Here's how the part is built. I have some questions about the finished solid (model axes, mm). Face numbers are marked on the shaded views. A direction names the side the tool comes from. Coordinates: 2 decimals unless noted, no trailing zeros. Order: outer loops, then holes, each group sorted by start corner. A loop starts at its lowest first (then second) coordinate and runs counter-clockwise, first axis right, second up. Notation, with made-up numbers: (-4, -3.5) - (37, -3.5) arc R20 cw to (37, 4.5) - close; hole circle Ø6 at (-20.5, -8.75). An arc over 180 degrees is marked (long way). Answer as CSV lines item,"result". Start each with the question number.
Item 1: Imagine slicing it at B-B on x = -207. List the corners of the cut face in (y, z) for me, and give its area (3 significant figures).
Item 2: Imagine slicing it at C-C on z = -2.75. List the corners of the cut face in (x, y) for me, and give its area (3 significant figures).
Item 3: I need wall thicknesses on line 1 (X direction, y = 90.75, z = -3.25); line 2 (Z direction, x = -208.5, y = 87.5); line 3 (Y direction, x = -190.5, z = -3.5). Which ranges of each line are inside material? Lowest first, please.
Item 4: Imagine slicing it at A-A on y = 87.5. List the corners of the cut face in (x, z) for me.
Item 5: Imagine slicing it at D-D on y = 91.25. List the corners of the cut face in (x, z) for me.
Item 6: On a 3-axis mill with a long thin cutter (end or side, diameter ignored), from which of +Z, -Z, +X, -X, +Y, -Y can I reach the whole of each face in a straight line? I mean the marked faces 1 and 2. Say none if no direction works.
Item 7: We'd pull the mould along X, two halves only. Please class the marked faces 3, 4 and 5: pulls with the +X half, pulls with the -X half, needs draft (parallel to the pull), parting line crosses it, or undercut.
Item 8: I'm going to push flat-ended pins straight in: pin 1 (1 mm diameter, centred on y = 90, z = 10.5, fed in from +X); pin 2 (5 mm diameter, centred on x = -194, y = 92, fed in from +Z). Where does each tip first touch, or does it pass through?
Autodesk Inventor part; units mm, degrees
ref_plane "YZ Plane" through (0, 0, 0) normal (1, 0, 0) x (0, 1, 0)
ref_plane "XZ Plane" through (0, 0, 0) normal (0, 1, 0) x (-1, 0, 0)
ref_plane "XY Plane" through (0, 0, 0) normal (0, 0, 1) x (1, 0, 0)
sketch "スケッチ1" plane through (0, 0, 0) normal (0, 0, 1) x (1, 0, 0)
  circle A0 centre (-137.47813, 108.715013) radius 1.5
  circle A1 centre (-137.47813, 108.715013) radius 4
  circle A2 centre (-84.833891, 108.084965) radius 1.5
  circle A3 centre (-84.833891, 108.084965) radius 4
  arc A4 (-118.947299, 71.123436) -> (-117.73095, 71.382243) centre (-118.502117, 72.018876) ccw
  arc A5 (-114.600271, 73.907195) -> (-117.73095, 71.382243) centre (-110, 65) ccw
  arc A6 (-114.600271, 73.907195) -> (-114.089743, 75.041147) centre (-115.059151, 74.795694) ccw
  line L0 (-114.089743, 75.041147) -> (-119.33341, 95.750821)
  arc A7 (-119.33341, 95.750821) -> (-120.080809, 96.480412) centre (-120.302818, 95.505368) ccw
  arc A8 (-121.730917, 97.23053) -> (-120.080809, 96.480412) centre (-119.081767, 100.868113) ccw
  arc A9 (-121.730917, 97.23053) -> (-122.772044, 97.31398) centre (-122.319616, 96.422178) ccw
  line L1 (-122.772044, 97.31398) -> (-145.176978, 85.94755)
  arc A10 (-145.176978, 85.94755) -> (-145.169733, 84.160308) centre (-144.724551, 85.055748) ccw
  line L2 (-145.169733, 84.160308) -> (-118.947299, 71.123436)
  arc A11 (-111.181518, 75.777506) -> (-110.19287, 75.023145) centre (-110.212109, 76.022959) ccw
  arc A12 (-100.681376, 68.696468) -> (-110.19287, 75.023145) centre (-110, 65) ccw
  arc A13 (-100.681376, 68.696468) -> (-99.603497, 68.076257) centre (-99.751838, 69.065193) ccw
  line L3 (-99.603497, 68.076257) -> (-77.042446, 71.460414)
  arc A14 (-77.042446, 71.460414) -> (-76.670938, 73.303609) centre (-77.190786, 72.449351) ccw
  line L4 (-76.670938, 73.303609) -> (-114.637331, 96.407596)
  arc A15 (-114.637331, 96.407596) -> (-116.126588, 95.307885) centre (-115.15718, 95.553338) ccw
  line L5 (-116.126588, 95.307885) -> (-111.181518, 75.777506)
  circle A16 centre (-150.294817, 85.033166) radius 1.5
  arc A17 (-124.129325, 99.989384) -> (-123.581755, 100.878808) centre (-124.581752, 100.881185) ccw
  arc A18 (-114.594354, 100.531773) -> (-123.581755, 100.878808) centre (-119.081767, 100.868113) ccw
  arc A19 (-114.594354, 100.531773) -> (-114.117, 99.602773) centre (-113.597151, 100.457031) ccw
  line L6 (-114.117, 99.602773) -> (-73.405222, 74.828115)
  arc A20 (-73.405222, 74.828115) -> (-72.36076, 74.831033) centre (-72.885373, 75.682374) ccw
  arc A21 (-73.660486, 68.382589) -> (-72.36076, 74.831033) centre (-70, 71) ccw
  arc A22 (-73.660486, 68.382589) -> (-74.622268, 68.789879) centre (-74.473928, 67.800942) ccw
  line L7 (-74.622268, 68.789879) -> (-99.158476, 65.109447)
  arc A23 (-99.158476, 65.109447) -> (-100.006948, 64.200283) centre (-99.010135, 64.120511) ccw
  arc A24 (-119.754961, 67.311137) -> (-100.006948, 64.200283) centre (-110, 65) ccw
  arc A25 (-119.754961, 67.311137) -> (-120.282843, 68.437115) centre (-120.728025, 67.541674) ccw
  line L8 (-120.282843, 68.437115) -> (-147.085218, 81.762313)
  arc A26 (-147.085218, 81.762313) -> (-148.083283, 81.700131) centre (-147.5304, 80.866873) ccw
  arc A27 (-148.11038, 88.384022) -> (-148.083283, 81.700131) centre (-150.294817, 85.033166) ccw
  arc A28 (-148.11038, 88.384022) -> (-147.111844, 88.329935) centre (-147.564271, 89.221736) ccw
  line L9 (-147.111844, 88.329935) -> (-124.129325, 99.989384)
  circle A29 centre (-110, 65) radius 7.025
  circle A30 centre (-119.081767, 100.868113) radius 1.5
  circle A31 centre (-70, 71) radius 1.5
  line L10 (-330.399972, 95) -> (-110, 65)
  circle A32 centre (-156.443214, 91.162336) radius 4
  circle A33 centre (-136.470623, 92.209055) radius 4
  line L11 (0, 0) -> (-155.794817, 0)
  line L12 (-329.051247, 104.90863) -> (-108.651275, 74.90863)
  circle A34 centre (-156.443214, 91.162336) radius 9
  circle A35 centre (-136.470623, 92.209055) radius 6
  line L13 (-156.443214, 91.162336) -> (-136.470623, 92.209055)
  circle A36 centre (-110, 65) radius 65
  circle A37 centre (-191.443214, 91.162336) radius 5
  line L14 (-191.443214, 91.162336) -> (-156.443214, 91.162336)
  line L15 (-191.443214, 91.162336) -> (-206.443214, 91.162336)
  circle A38 centre (-206.443214, 91.162336) radius 5
  line L16 (-206.443214, 91.162336) -> (-221.443214, 91.162336)
  circle A39 centre (-221.443214, 91.162336) radius 5
  line L17 (-221.443214, 91.162336) -> (-236.443214, 91.162336)
  circle A40 centre (-236.443214, 91.162336) radius 5
  line L18 (-206.843214, 96.14631) -> (-157.163214, 100.133489)
  line L19 (-206.843214, 86.178361) -> (-157.163214, 82.191182)
  line L20 (-135.882319, 98.180143) -> (-155.560758, 100.118968)
  line L21 (-154.629369, 82.34701) -> (-135.261393, 86.332171)
  circle A41 centre (-206.443214, 91.162336) radius 1.5
  circle A42 centre (-191.443214, 91.162336) radius 1.5
  line L22 (-236.443214, 91.162336) -> (-191.443214, 91.162336) construction
  line L23 (-236.443214, 86.162336) -> (-191.443214, 86.162336)
  line L24 (-191.443214, 96.162336) -> (-236.443214, 96.162336)
  arc A43 (-236.443214, 96.162336) -> (-236.443214, 86.162336) centre (-236.443214, 91.162336) ccw
  arc A44 (-191.443214, 86.162336) -> (-191.443214, 96.162336) centre (-191.443214, 91.162336) ccw
  point P0 (-202.811763, 87.725395)
  point P1 (-169.324077, 83.167179)
  point P2 (-153.510113, 82.653698)
  point P3 (-153.460125, 82.587594)
  point P4 (-191.336809, 86.163468)
  point P5 (-192.881846, 86.373772)
  point P6 (-213.943214, 91.162336)
  dimension "d0" = 8
  dimension "d1" = 8
  dimension "d2" = 95
  dimension "d3" = 7.75125
  dimension "d4" = 10
  dimension "d5" = 18
  dimension "d6" = 12
  dimension "d7" = 20
  dimension "d8" = 3
  dimension "d9" = 130
  dimension "d10" = 10
  dimension "d11" = 35
  dimension "d12" = 15
  dimension "d13" = 10
  dimension "d14" = 15
  dimension "d15" = 10
  dimension "d16" = 15
  dimension "d17" = 10
  dimension "d18" = 3
  dimension "d19" = 3
  dimension "d20" = 10
extrude "押し出し1" add sketch "スケッチ1" against normal blind 5 contours A37 L12 | L12 A37 L15 A42 L14 | L23 A39 L12 A38 L19 | L19 A38 L23 | A37 L23 A38 L12 | L12 A38 L15 A37 | L14 A42 L15 A37 | A38 L12 | L23 A40 L17 L12 A39 | A39 L12 | L12 A38 L16 A41 L15 | L15 A38 L24 A37 | A42 L15 L14 | L14 L15 A42 | L24 A38 L18 | L18 A38 L16 A39 L24 | L12 A39 L16 A38 | A39 L17 L16 L12 | L12 L17 A39 | L15 A41 L16 A38 | A39 L16 L17 | A39 L17 L12 A40 L24 | L17 A40 L12 | A41 L16 L15 | L15 L16 A41
hole "穴1" at (-206.443214, 91.162336, 0) at (-191.443214, 91.162336, 0) direction (0, 0, -1) diameter 3 depth 12 tip angle 118
sketch "スケッチ2" plane through (0, 0, 0) normal (0, 0, 1) x (1, 0, 0)
  circle A0 centre (-206.443214, 91.162336) radius 1.5
  circle A1 centre (-191.443214, 91.162336) radius 1.5
  line L0 (-236.443214, 96.162336) -> (-191.443214, 96.162336)
  arc A2 (-191.443214, 86.162336) -> (-191.443214, 96.162336) centre (-191.443214, 91.162336) ccw
  line L1 (-191.443214, 86.162336) -> (-236.443214, 86.162336)
  arc A3 (-236.443214, 96.162336) -> (-236.443214, 86.162336) centre (-236.443214, 91.162336) ccw
  line L2 (-236.443214, 96.162336) -> (-239.443214, 96.162336)
  line L3 (-239.443214, 96.162336) -> (-239.443214, 86.162336)
  line L4 (-191.443214, 86.162336) -> (-236.443214, 86.162336)
  line L5 (-239.443214, 86.162336) -> (-236.443214, 86.162336)
  arc A4 (-191.443214, 86.162336) -> (-191.443214, 96.162336) centre (-191.443214, 91.162336) ccw
  line L6 (-191.443214, 96.162336) -> (-186.443214, 96.162336)
  line L7 (-186.443214, 96.162336) -> (-186.443214, 86.162336)
  line L8 (-186.443214, 86.162336) -> (-191.443214, 86.162336)
  line L9 (-191.443214, 96.162336) -> (-236.443214, 96.162336)
  line L10 (-236.443214, 86.162336) -> (-191.443214, 86.162336)
  arc A5 (-236.443214, 96.162336) -> (-236.443214, 86.162336) centre (-236.443214, 91.162336) ccw
  circle A6 centre (-234.443214, 91.162336) radius 5
  circle A7 centre (-219.443214, 91.162336) radius 5
  circle A8 centre (-206.443214, 91.162336) radius 1.5
  circle A9 centre (-206.443214, 91.162336) radius 5
  point P0 (0, 0)
  point P1 (-239.443214, 87.162336)
  point P2 (-186.443214, 91.162336)
  point P3 (-239.443214, 87.162336)
  point P4 (-239.443214, 95.162336)
  point P5 (-234.443214, 86.162336)
  point P6 (-234.443214, 96.162336)
  point P7 (-239.443214, 95.162336)
  dimension "d32" = 53
  dimension "d33" = 10
  dimension "d34" = 10
  dimension "d35" = 15
  dimension "d36" = 15
  dimension "d46" = 10
extrude "押し出し2" add sketch "スケッチ2" against normal blind 5 contours L0 A6 L3 A3 | A3 L3 L2 | A6 | A6 L1 A3 L3 | A3 L5 L3 | L6 L7 A2 | L7 L8 A2
hole "穴2" at (-234.443214, 91.162336, 0) at (-219.443214, 91.162336, 0) direction (0, 0, -1) diameter 3 depth 12 tip angle 118
sketch "スケッチ3" plane through (0, 0, 0) normal (0, 0, 1) x (1, 0, 0)
  circle A0 centre (-219.443214, 91.162336) radius 1.5
  line L0 (-186.443214, 96.162336) -> (-186.443214, 86.162336)
  line L1 (-186.443214, 86.162336) -> (-239.443214, 86.162336)
  line L2 (-239.443214, 86.162336) -> (-239.443214, 96.162336)
  line L3 (-239.443214, 96.162336) -> (-186.443214, 96.162336)
  circle A1 centre (-206.443214, 91.162336) radius 1.5
  circle A2 centre (-191.443214, 91.162336) radius 1.5
  line L4 (-186.443214, 96.162336) -> (-239.443214, 96.162336)
  line L5 (-212.943214, 96.162336) -> (-212.943214, 86.162336)
  line L6 (-239.443214, 86.162336) -> (-186.443214, 86.162336)
  circle A3 centre (-234.443214, 91.162336) radius 1.5
  point P0 (0, 0)
bend part "曲げパーツ1" radius 1 angle 30.54 line through (-212.943214, 96.162336, 0) along (0, -1, 0) centre toward (0, 0, 1) moving side (-1, 0, 0) both sides no
equation "\"d36\" = d35"
properties part number "カウンター 取り付け根元曲げパーツ" material "アルミニウム 6061"
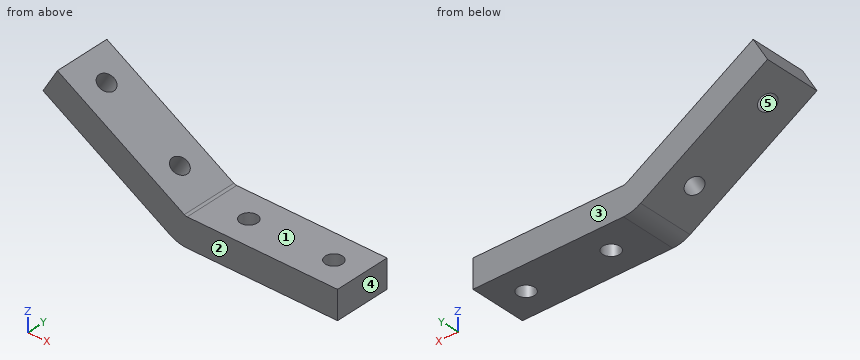
Responses:
1,outline,"(86.16, -5) - (89.77, -5) - (89.77, 0) - (86.16, 0) - close; (92.56, -5) - (96.16, -5) - (96.16, 0) - (92.56, 0) - close"
1,area,"36.1 mm^2"
2,outline,"(-218.39, 86.16) - (-186.44, 86.16) - (-186.44, 96.16) - (-218.39, 96.16) - close; hole circle Ø3 at (-206.44, 91.16); hole circle Ø3 at (-191.44, 91.16)"
2,area,"305 mm^2"
3,line 1,"x = -217.55 to -207.89, -205 to -192.89, -190 to -186.44"
3,line 2,"z = -5 to 0"
3,line 3,"y = 86.16 to 90, 92.33 to 96.16"
4,outline,"(-238.36, 9.03) - (-215.99, -4.17) arc R6 ccw to (-212.94, -5) - (-186.44, -5) - (-186.44, 0) - (-212.94, 0) arc R1 cw to (-213.45, 0.14) - (-235.82, 13.33) - close"
5,outline,"(-238.36, 9.03) - (-235.34, 7.25) - (-232.8, 11.55) - (-235.82, 13.33) - close; (-232.76, 5.73) - (-222.42, -0.37) - (-219.88, 3.93) - (-230.22, 10.03) - close; (-219.84, -1.9) - (-215.99, -4.17) arc R6 ccw to (-212.94, -5) - (-207.94, -5) - (-207.94, 0) - (-212.94, 0) arc R1 cw to (-213.45, 0.14) - (-217.3, 2.41) - close; (-204.95, -5) - (-192.94, -5) - (-192.94, 0) - (-204.95, 0) - close; (-189.95, -5) - (-186.44, -5) - (-186.44, 0) - (-189.95, 0) - close"
6,face 1,"+Z, +X, +Y, -Y"
6,face 2,"+Z, -Z, +X, -X, -Y"
7,face 3,"needs draft"
7,face 4,"pulls with the +X half"
7,face 5,"undercut"
8,pin 1,"stops at x = -230.17"
8,pin 2,"stops at z = 0"
